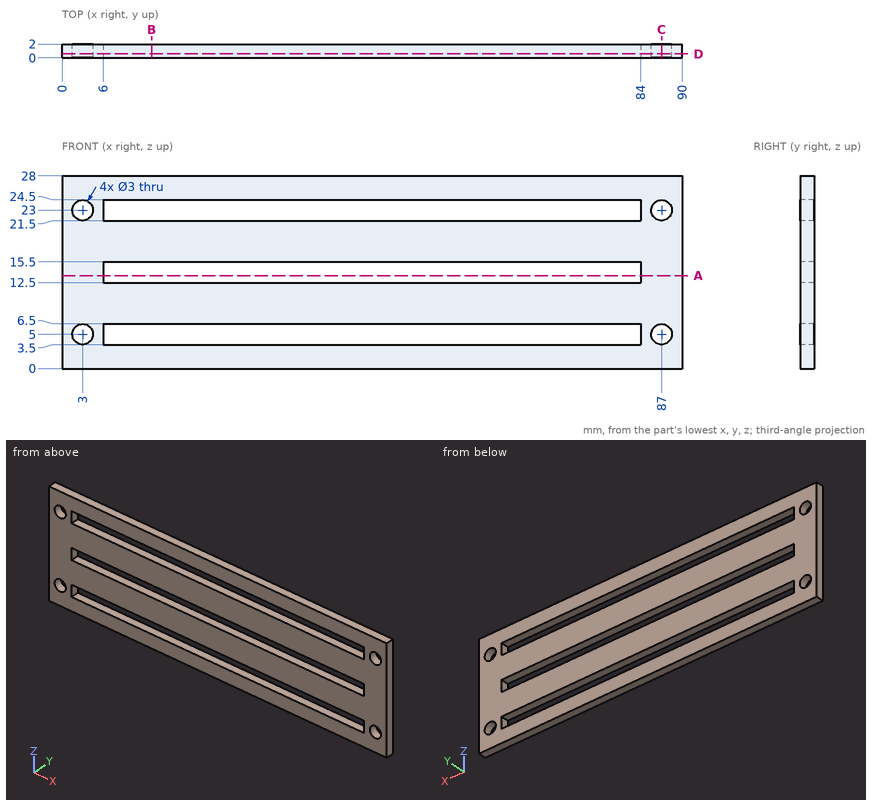
Answer from the drawing. Dimensions are ordinates in mm from the lowest x, y and z of the part. Round coordinates to 2 decimals unless told otherwise and drop trailing zeros. Order: outer loops, then holes, each group sorted by start corner. A loop starts at its lowest first (then second) coordinate and runs counter-clockwise, first axis right, second up. Notation, with made-up numbers: (-10, 63.25) - (18, 63.25) arc R27 cw to (18, 100.25) - close; hole circle Ø11 at (88.25, 43). An arc over 180 degrees is marked (long way). Put each result on its own line as item: value. Start each with the question number.
(1) Find section A-A (z = 13.5). Give the vertices of the cut face in (x, y), plus the area to 3 significant figures.
(2) Find section D-D (y = 0.55). Give the vertices of the cut face in (x, z), plus the area to 3 significant figures.
(3) Find section C-C (x = 87). Give the vertices of the cut face in (y, z), plus the area to 3 significant figures.
(4) Find section B-B (x = 13). Give the vertices of the cut face in (y, z), plus the area to 3 significant figures.
(5) Given P1, Ø2.5, axis at x = 87, z = 5, coming from the +Y side, flat-ended and moving along its own axis, determine where the tip first touches the part or whether it passes through.
(6) Straight lines are drawn through the part: probe 1 along Z at (x, y) = (74.5, 1.15); probe 2 along X at (y, z) = (1.6, 5); probe 3 along Z at (x, y) = (87, 1.25). For each, find the intervals that lie inside material, in ascending order. Write a range as from..to.
Reply:
1. outline: (0, 0) - (6, 0) - (6, 2) - (0, 2) - close; (84, 0) - (90, 0) - (90, 2) - (84, 2) - close
1. area: 24.0 mm^2
2. outline: (0, 0) - (90, 0) - (90, 28) - (0, 28) - close; hole circle Ø3 at (3, 5); hole circle Ø3 at (3, 23); hole (6, 3.5) - (84, 3.5) - (84, 6.5) - (6, 6.5) - close; hole (6, 12.5) - (84, 12.5) - (84, 15.5) - (6, 15.5) - close; hole (6, 21.5) - (84, 21.5) - (84, 24.5) - (6, 24.5) - close; hole circle Ø3 at (87, 5); hole circle Ø3 at (87, 23)
2. area: 1,790 mm^2
3. outline: (0, 0) - (2, 0) - (2, 3.5) - (0, 3.5) - close; (0, 6.5) - (2, 6.5) - (2, 21.5) - (0, 21.5) - close; (0, 24.5) - (2, 24.5) - (2, 28) - (0, 28) - close
3. area: 44.0 mm^2
4. outline: (0, 0) - (2, 0) - (2, 3.5) - (0, 3.5) - close; (0, 6.5) - (2, 6.5) - (2, 12.5) - (0, 12.5) - close; (0, 15.5) - (2, 15.5) - (2, 21.5) - (0, 21.5) - close; (0, 24.5) - (2, 24.5) - (2, 28) - (0, 28) - close
4. area: 38.0 mm^2
5. P1: through
6. probe 1: 0..3.5, 6.5..12.5, 15.5..21.5, 24.5..28
6. probe 2: 0..1.5, 4.5..6, 84..85.5, 88.5..90
6. probe 3: 0..3.5, 6.5..21.5, 24.5..28
